Input: part model. Units: mm. Frame: model coordinates. Round coordinates to 2 decimals unless told otherwise and drop trailing zeros. Loops run counter-clockwise (first coordinate to the right, second up) from the corner with the lowest first, then second, coordinate; pieces in that order, holes last. Notation, with made-up numbers: (86, 82) - (107, 82) arc R21 ccw to (107, 86) - close; hole circle Ø8 at (29.25, 42.5). An arc over 180 degrees is marked (long way). One line per question, with ' | ' between items. Start each with the question number.
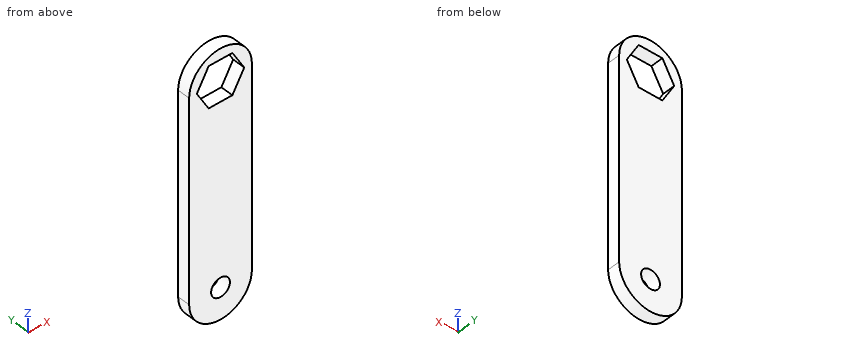
from build123d import *

# Parameters (mm, degrees)
SKETCH_1_R      = 1.5
EXTRUDE_1_DEPTH = 2


with BuildPart() as part:
    # 草图1 → 凸台-拉伸1 (new body)
    with BuildSketch(Plane(origin=(0, 0, 0), x_dir=(1, 0, 0), z_dir=(0, 1, 0))):
        with BuildLine():
            Line((-5, -16), (-5, 16))
            ThreePointArc((-5, 16), (0, 21), (5, 16))
            Line((5, 16), (5, -16))
            ThreePointArc((5, -16), (0, -21), (-5, -16))
        make_face()
        with Locations(Location((0, 16, 0), (0, 0, 270))):
            Circle(SKETCH_1_R, mode=Mode.SUBTRACT)
        Polygon((1.890822132, -12.725), (-1.890822132, -12.725), (-3.781644263, -16), (-1.890822132, -19.275), (1.890822132, -19.275), (3.781644263, -16), align=None, mode=Mode.SUBTRACT)
    extrude(amount=EXTRUDE_1_DEPTH)


solid = part.part
(1) Section A-A, the plane x = 0. Output: boundary loops of the cut face in (y, z) (3 decimals), plus the area to 3 significant figures.
(2) Line query: line 1 along X through (y, z) = (0.5, -16); line 2 along Z through (x, y) = (2, 0.15); line 3 along Z through (x, y) = (-3.5, 1). Output: solid intervals per line, ascending. Write a range as from..to.
(3) Section C-C, the plane z = 13.5. Output: boundary loops of the cut face in (x, y).
(4) Pin query (flat end, axial travel): P1, Ø1, axis at x = 1, y = 1.5, coming from the +Z side. Return the tip coordinate at first contact, or that it passes through.
(5) Section B-B, the plane y = 1.2. Output: boundary loops of the cut face in (x, z) (3 decimals), plus the area to 3 significant figures.
(6) Section D-D, the plane x = 2.75. Output: boundary loops of the cut face in (y, z), plus the area to 3 significant figures.
Derived:
1) outline: (0, -21) - (2, -21) - (2, -17.5) - (0, -17.5) - close; (0, -14.5) - (2, -14.5) - (2, 12.725) - (0, 12.725) - close; (0, 19.275) - (2, 19.275) - (2, 21) - (0, 21) - close | area: 64.9 mm²
2) line 1: x = -5..-1.5, 1.5..5 | line 2: z = -20.58..12.91, 19.09..20.58 | line 3: z = -19.57..15.51, 16.49..19.57
3) outline: (-5, 0) - (-2.34, 0) - (-2.34, 2) - (-5, 2) - close; (2.34, 0) - (5, 0) - (5, 2) - (2.34, 2) - close
4) P1: stops at z = 20.97
5) outline: (-5, -16) arc R5 ccw to (5, -16) - (5, 16) arc R5 ccw to (-5, 16) - close; hole (-3.782, 16) - (-1.891, 12.725) - (1.891, 12.725) - (3.782, 16) - (1.891, 19.275) - (-1.891, 19.275) - close; hole circle Ø3 at (0, -16) | area: 354 mm²
6) outline: (0, -20.18) - (2, -20.18) - (2, 14.21) - (0, 14.21) - close; (0, 17.79) - (2, 17.79) - (2, 20.18) - (0, 20.18) - close | area: 73.6 mm²
